Verification items for the finished model (mm, model axes). A direction names the side the tool comes from. Coordinates: 2 decimals unless noted, no trailing zeros. Loops run counter-clockwise (first coordinate to the right, second up) from the corner with the lowest first, then second, coordinate; pieces in that order, holes last. Notation, with made-up numbers: (85.5, -26) -> (106.5, -26) arc R30 cw to (106.5, 1) -> close; hole circle Ø4 at (70, 63.5). An arc over 180 degrees is marked (long way). Use CSV: the item, a comma, the result in double quotes. Start each with the question number.
Autodesk Inventor part; units mm, degrees
ref_plane "YZ Plane" through (0, 0, 0) normal (1, 0, 0) x (0, 1, 0)
ref_plane "XZ Plane" through (0, 0, 0) normal (0, 1, 0) x (-1, 0, 0)
ref_plane "XY Plane" through (0, 0, 0) normal (0, 0, 1) x (1, 0, 0)
sketch "Sketch1" plane through (0, 0, 0) normal (0, 0, 1) x (1, 0, 0)
  line L0 (100, 100) -> (-100, 100)
  line L1 (-100, 100) -> (-100, -100)
  line L2 (-100, -100) -> (100, -100)
  line L3 (100, -100) -> (100, 100)
  line L4 (100, 100) -> (-100, -100) construction
  line L5 (-100, 100) -> (100, -100) construction
  point P0 (0, 0)
  dimension "d0" = 200
  dimension "d1" = 200
extrude "Extrusion1" add sketch "Sketch1" along normal blind 3
fillet "Fillet1" radius 5 4 edges at (100, 100, 1.5) (-100, 100, 1.5) (100, -100, 1.5) (-100, -100, 1.5)
sketch "Sketch2" plane through (0, 0, 3) normal (0, 0, 1) x (1, 0, 0)
  circle A0 centre (0, 0) radius 2.55
  dimension "d5" = 5.1
extrude "Extrusion2" cut sketch "Sketch2" against normal blind 10
sketch "Sketch3" plane through (0, 0, 3) normal (0, 0, 1) x (1, 0, 0)
  circle A0 centre (0, 0) radius 4.75
  dimension "d10" = 9.5
extrude "Extrusion3" cut sketch "Sketch3" against normal blind 0.7
sketch "Sketch4" plane through (0, 0, 0) normal (0, 0, -1) x (-1, 0, 0)
  point P0 (0, 0)
sketch "Sketch5" plane through (0, 0, 0) normal (0, 0, -1) x (-1, 0, 0)
  point P0 (0, 0)
sketch "Sketch6" plane through (0, 0, 0) normal (0, 0, -1) x (-1, 0, 0)
  circle A0 centre (-77, 76.9998) radius 6
  line L0 (-93.7439, 99.9999) -> (-93.7439, -0.0001)
  line L1 (-93.7439, -0.0001) -> (78.7368, -0.0001)
  circle A1 centre (-77, -77) radius 6
  line L2 (95, -100) -> (-95, -100)
  line L3 (0, -100) -> (0, 48.6306)
  circle A2 centre (77, 76.9998) radius 6
  circle A3 centre (77, -77) radius 6
  line L4 (-100, -95) -> (-100, 95)
  point P0 (0, 0)
  point P1 (-93.7439, 89.8675)
  point P2 (-93.7439, 85.1564)
  dimension "d11" = 12
  dimension "d13" = 100
  dimension "d22" = 23
  dimension "d23" = 23
extrude "Extrusion4" cut sketch "Sketch6" against normal blind 10
sketch "Sketch8" plane through (0, 0, 0) normal (0, 0, -1) x (-1, 0, 0)
  circle A0 centre (0, 0) radius 4.24
  dimension "d19" = 8.48
extrude "Extrusion6" cut sketch "Sketch8" against normal blind 0.5
sketch "Sketch9" plane through (0, 0, 3) normal (0, 0, 1) x (1, 0, 0)
  circle A0 centre (-77, -77) radius 6
  circle A1 centre (-77, -77) radius 5
  circle A2 centre (77, -77) radius 6
  circle A3 centre (77, -77) radius 5
  circle A4 centre (77, 76.9998) radius 6
  circle A5 centre (77, 76.9998) radius 5
  circle A6 centre (-77, 76.9998) radius 6
  circle A7 centre (-77, 76.9998) radius 5
  point P0 (0, 0)
  dimension "d24" = 10
  dimension "d25" = 10
  dimension "d26" = 10
  dimension "d27" = 10
extrude "Extrusion7" add sketch "Sketch9" against normal blind 0.5
properties part number "Plate" material "Aluminum 6061"
1. Cross-section at A-A, the plane x = -77. Record the boundary of the cut face in (y, z).
2. Scan lines: line 1 (Y direction, x = 77, z = 1.6); line 2 (Y direction, x = -77, z = 2.6); line 3 (Y direction, x = 0, z = 0.2). Record each from-to range of solid material in increasing order.
3. Depth check by flat-ended pin: pin 1 (9.5 mm diameter, centred on x = 75.5, y = 79.5, fed in from -Z); pin 2 (9.5 mm diameter, centred on x = -76, y = 77.5, fed in from -Z); pin 3 (3 mm diameter, centred on x = 2, y = 0.5, fed in from +Z); pin 4 (7 mm diameter, centred on x = 0, y = 0, fed in from -Z). Enter the tip coordinate at first touch or a pass-through.
4. Cross-section at C-C, the plane x = 0. Record the boundary of the cut face in (y, z), plus the area to 3 significant figures.
5. Set-up check for faces 4 (the cylindrical face through (-4.044, 1.274, 0.246)), 5 (the flat face through (2, -2, 2.3)), 6 (the cylindrical face through (81.619, -78.915, 2.754)): record each of +Z, -Z, +X, -X, +Y, -Y from which the full face is reachable in a straight line by a thin tool's end or side.
6. Release check for a two-part mould opening along X. For faces 1 (the cylindrical face through (-74.312, 81.216, 2.754)), 2 (the flat face through (-1, 24, 3)), 3 (the cylindrical face through (-99, -98, 2)) record: released by +X, released by -X, zero draft, split by the parting line, or undercut.
Solution:
1,outline,"(-100, 0) -> (-83, 0) -> (-83, 2.5) -> (-82, 2.5) -> (-82, 3) -> (-100, 3) -> close; (-72, 2.5) -> (-71, 2.5) -> (-71, 0) -> (71, 0) -> (71, 2.5) -> (72, 2.5) -> (72, 3) -> (-72, 3) -> close; (82, 2.5) -> (83, 2.5) -> (83, 0) -> (100, 0) -> (100, 3) -> (82, 3) -> close"
2,line 1,"y = -100 to -83, -71 to 71, 83 to 100"
2,line 2,"y = -100 to -82, -72 to 72, 82 to 100"
2,line 3,"y = -100 to -4.24, 4.24 to 100"
3,pin 1,"stops at z = 0"
3,pin 2,"stops at z = 2.5"
3,pin 3,"stops at z = 2.3"
3,pin 4,"stops at z = 0.5"
4,outline,"(-100, 0) -> (-4.24, 0) -> (-4.24, 0.5) -> (-2.55, 0.5) -> (-2.55, 2.3) -> (-4.75, 2.3) -> (-4.75, 3) -> (-100, 3) -> close; (2.55, 0.5) -> (4.24, 0.5) -> (4.24, 0) -> (100, 0) -> (100, 3) -> (4.75, 3) -> (4.75, 2.3) -> (2.55, 2.3) -> close"
4,area,"580 mm2"
5,face 4,"-Z"
5,face 5,"+Z"
5,face 6,"+Z, -Z"
6,face 1,"undercut"
6,face 2,"zero draft"
6,face 3,"released by -X"
